Geometry check sheet. Reference: the model listing, model coordinates, mm. A direction names the side the tool comes from. Round coordinates to 2 decimals unless told otherwise and drop trailing zeros. Put each result on its own line as item: value. Start each with the question number.
(1) Material ranges on probe 1 along X at (y, z) = (16.5, 1.65); probe 2 along Y at (x, z) = (-90, 2.7); probe 3 along X at (y, z) = (11.5, 2), recorded low to high.
(2) Tool access check on faces 1 (the cylindrical face through (-7.64, 30.86, 1.51)), 2 (the flat face through (-25.135, 7, 2)), 3 (the flat face through (-119.38, 1, 2)). Record the directions out of +Z, -Z, +X, -X, +Y, -Y that give a thin tool (end or side, any length) a straight path to the whole face; none if there is none.
(3) Gauge pin test, flat ends, axial feed: pin 1 (1.5 mm diameter, centred on y = 1, z = 1.5, fed in from -X); pin 2 (0.8 mm diameter, centred on x = -90, z = 2, fed in from -Y). Record the tip position at first contact, or that the pin passes through.
from build123d import *

# Parameters (mm, degrees)
BOSS_EXTRUDE2_DEPTH = 2.9718
SKETCH4_W           = 12.7
SKETCH4_H           = 2.972153091
CUT_EXTRUDE1_DEPTH  = 2.9718
CUT_EXTRUDE2_DEPTH  = 2.9718
FILLET1_R           = 25.4


with BuildPart() as part:
    # Sketch2 → Boss-Extrude2 (new body)
    with BuildSketch(Plane.XY):
        with BuildLine():
            Line((-190.5, 0), (0, 0))
            Line((0, 0), (0, 38.1))
            Line((0, 38.1), (-125.518660072, 38.1))
            add(Edge.make_bspline(
                [(-125.518660072, 38.1), (-137.686277491, 3.422332996), (-190.5, 0)],
                knots=[0, 0, 0, 1, 1, 1], degree=2))
        make_face()
    extrude(amount=BOSS_EXTRUDE2_DEPTH)

    # Sketch4 → Cut-Extrude1 (cut)
    with BuildSketch(Plane.XY.offset(2.9718)):
        with Locations((-26.67, 1.486076546)):
            Rectangle(SKETCH4_W, SKETCH4_H)
        with Locations((-59.69, 1.486076546)):
            Rectangle(SKETCH4_W, SKETCH4_H)
        with Locations((-92.71, 1.486076546)):
            Rectangle(SKETCH4_W, SKETCH4_H)
        with BuildLine():
            add(Edge.make_bspline(
                [(-169.427921187, 2.972153091), (-179.000448456, 0.745171762), (-190.5, 0)],
                knots=[0.782262052, 0.782262052, 0.782262052, 1, 1, 1], degree=2))
            Line((-190.5, 0), (-119.38, 0))
            Line((-119.38, 0), (-119.38, 2.972153091))
            Line((-119.38, 2.972153091), (-169.427921187, 2.972153091))
        make_face()
    extrude(amount=-CUT_EXTRUDE1_DEPTH, mode=Mode.SUBTRACT)

    # Sketch5 → Cut-Extrude2 (cut)
    with BuildSketch(Plane.XY.offset(2.9718)):
        Polygon((-91.313, 14.402153091), (-91.313, 18.212153091), (-94.107, 18.212153091), (-94.107, 14.402153091), (-95.758, 14.402153091), (-95.758, 12.116153091), (-94.244804958, 12.116153091), (-94.244804958, 2.972153091), (-91.175195042, 2.972153091), (-91.175195042, 12.116153091), (-89.662, 12.116153091), (-89.662, 14.402153091), align=None)
        Polygon((-58.293, 14.402153091), (-58.293, 18.212153091), (-61.087, 18.212153091), (-61.087, 14.402153091), (-62.738, 14.402153091), (-62.738, 12.116153091), (-61.224804958, 12.116153091), (-61.224804958, 2.972153091), (-58.155195042, 2.972153091), (-58.155195042, 12.116153091), (-56.642, 12.116153091), (-56.642, 14.402153091), align=None)
        Polygon((-26.67, 2.972153091), (-26.67, 18.212153091), (-28.067, 18.212153091), (-28.067, 14.402153091), (-29.718, 14.402153091), (-29.718, 12.116153091), (-28.204804958, 12.116153091), (-28.204804958, 2.972153091), align=None)
        Polygon((-25.273, 18.212153091), (-26.67, 18.212153091), (-26.67, 2.972153091), (-25.135195042, 2.972153091), (-25.135195042, 12.116153091), (-23.622, 12.116153091), (-23.622, 14.402153091), (-25.273, 14.402153091), align=None)
    extrude(amount=-CUT_EXTRUDE2_DEPTH, mode=Mode.SUBTRACT)

    # Fillet1
    fillet1_edges = [part.edges().sort_by_distance(p)[0] for p in [
        (0, 38.1, 1.4859),
    ]]
    fillet(fillet1_edges, radius=FILLET1_R)


solid = part.part
Answers follow:
1. probe 1: x = -140.34 to -94.11, -91.31 to -61.09, -58.29 to -28.07, -25.27 to -0.29
1. probe 2: y = 2.97 to 12.12, 14.4 to 38.1
1. probe 3: x = -147.4 to -94.24, -91.18 to -61.22, -58.16 to -28.2, -25.14 to 0
2. face 1: +Z, -Z, +X, +Y
2. face 2: +Z, -Z, -Y
2. face 3: +Z, -Z, -X, -Y
3. pin 1: stops at x = -119.38
3. pin 2: stops at y = 2.97
